Build history of the part. All positions in model axes, mm. Face numbers are marked on the shaded views. A direction names the side the tool comes from. Round coordinates to 2 decimals unless told otherwise and drop trailing zeros. Order: outer loops, then holes, each group sorted by start corner. A loop starts at its lowest first (then second) coordinate and runs counter-clockwise, first axis right, second up. Notation, with made-up numbers: (42, 38) -> (97, 38) arc R34 cw to (97, 73) -> close; hole circle Ø10 at (17, 19). An arc over 180 degrees is marked (long way). Write item = value, one per line.
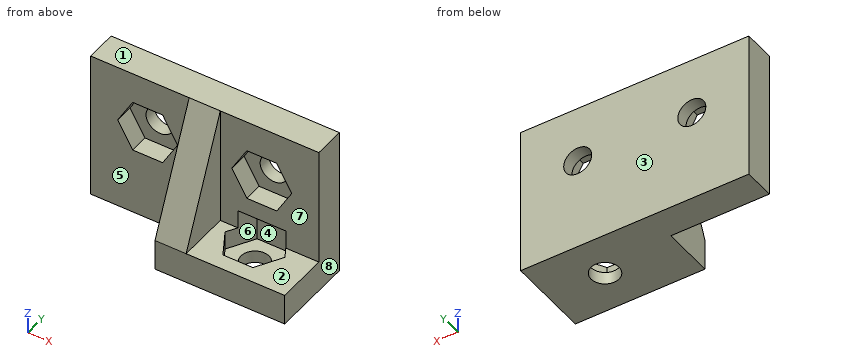
from build123d import *

# Parameters (mm, degrees)
EXTRUDE003_DEPTH  = 3.6
CYLINDER002_R     = 1.35
CYLINDER002_DEPTH = 3
EXTRUDE002_DEPTH  = 1.8
CYLINDER003_R     = 1.35
CYLINDER003_DEPTH = 30
EXTRUDE001_DEPTH  = 1.8
CYLINDER_R        = 1.35
CYLINDER_DEPTH    = 3
BOX_W             = 22
BOX_H             = 3
BOX_DEPTH         = 14.5
BOX001_W          = 12.5
BOX001_H          = 5
BOX001_DEPTH      = 3
EXTRUDE_DEPTH     = 3


with BuildPart() as extrude003:
    # Sketch003 → Extrude003 (new body)
    with BuildSketch(Plane.XY):
        Polygon((2.8868, 0), (1.4434, 2.500042), (-1.4434, 2.500042), (-2.8868, 0), (-1.4434, -2.500042), (1.4434, -2.500042), align=None)
    extrude(amount=EXTRUDE003_DEPTH)


with BuildPart() as extrude003_1:
    # Extrude003 placement: moved
    add(extrude003.part.moved(Location((16.5, -1, 1.2))))


with BuildPart() as hole03:
    # Cylinder002 → Cylinder002 (new body)
    with BuildSketch(Plane(origin=(16.5, -1, 0), x_dir=(0, 1, 0), z_dir=(0, 0, 1))):
        Circle(CYLINDER002_R)
    extrude(amount=CYLINDER002_DEPTH)

    # Fusion002: union Extrude003
    add(extrude003_1.part)


with BuildPart() as extrude002:
    # Sketch002 → Extrude002 (new body)
    with BuildSketch(Plane(origin=(16.5, 1.8, 9), x_dir=(1, 0, 0), z_dir=(0, -1, 0))):
        Polygon((2.8868, 0), (1.4434, 2.500042), (-1.4434, 2.500042), (-2.8868, 0), (-1.4434, -2.500042), (1.4434, -2.500042), align=None)
    extrude(amount=EXTRUDE002_DEPTH)


with BuildPart() as hole02:
    # Cylinder003 → Cylinder003 (new body)
    with BuildSketch(Plane(origin=(16.5, 3, 9), x_dir=(1, 0, 0), z_dir=(0, -1, 0))):
        Circle(CYLINDER003_R)
    extrude(amount=CYLINDER003_DEPTH)

    # Fusion001: union Extrude002
    add(extrude002.part)


with BuildPart() as extrude001:
    # Sketch001 → Extrude001 (new body)
    with BuildSketch(Plane(origin=(5.5, 1.8, 9), x_dir=(1, 0, 0), z_dir=(0, -1, 0))):
        Polygon((2.8868, 0), (1.4434, 2.500042), (-1.4434, 2.500042), (-2.8868, 0), (-1.4434, -2.500042), (1.4434, -2.500042), align=None)
    extrude(amount=EXTRUDE001_DEPTH)


with BuildPart() as hole01:
    # Cylinder → Cylinder (new body)
    with BuildSketch(Plane(origin=(5.5, 3, 9), x_dir=(1, 0, 0), z_dir=(0, -1, 0))):
        Circle(CYLINDER_R)
    extrude(amount=CYLINDER_DEPTH)

    # Fusion: union Extrude001
    add(extrude001.part)


with BuildPart() as cut001:
    # Box → Box (new body)
    with BuildSketch(Plane.XY):
        with Locations((11, 1.5)):
            Rectangle(BOX_W, BOX_H)
    extrude(amount=BOX_DEPTH)

    # Cut: cut Hole01
    add(hole01.part, mode=Mode.SUBTRACT)

    # Cut001: cut Hole02
    add(hole02.part, mode=Mode.SUBTRACT)


with BuildPart() as cut002:
    # Box001 → Box001 (new body)
    with BuildSketch(Plane(origin=(9.5, -5, 0), x_dir=(1, 0, 0), z_dir=(0, 0, 1))):
        with Locations((6.25, 2.5)):
            Rectangle(BOX001_W, BOX001_H)
    extrude(amount=BOX001_DEPTH)

    # Fusion003: union Cut001
    add(cut001.part)

    # Cut002: cut Hole03
    add(hole03.part, mode=Mode.SUBTRACT)


with BuildPart() as left_hand_bracket:
    # Sketch → Extrude (new body)
    with BuildSketch(Plane(origin=(0, 0, 1.4), x_dir=(0, 1, 0), z_dir=(1, 0, 0))):
        Polygon((0, 11.5), (0, 0), (-5, 0), align=None)
    extrude(amount=EXTRUDE_DEPTH)


with BuildPart() as left_hand_bracket_1:
    # Extrude placement: moved
    add(left_hand_bracket.part.moved(Location((9.5, 0, 1.6))))

    # Fusion004: union Cut002
    add(cut002.part)


solid = left_hand_bracket_1.part
Q1. Cut at C-C, the plane x = 16.5. List the corners of the cut face in (y, z), and give its area (3 significant figures).
Check values:
outline = (-5, 0) -> (-2.35, 0) -> (-2.35, 1.2) -> (-3.5, 1.2) -> (-3.5, 3) -> (-5, 3) -> close; (0, 4.8) -> (1.5, 4.8) -> (1.5, 1.2) -> (0.35, 1.2) -> (0.35, 0) -> (3, 0) -> (3, 7.65) -> (1.8, 7.65) -> (1.8, 6.5) -> (0, 6.5) -> close; (0, 11.5) -> (1.8, 11.5) -> (1.8, 10.35) -> (3, 10.35) -> (3, 14.5) -> (0, 14.5) -> close
area = 31.3 mm²
Q2. Cut at A-A, the plane x = 5.5. List the corners of the cut face in (y, z), and give its area (3 significant figures).
Check values:
outline = (0, 0) -> (3, 0) -> (3, 7.65) -> (1.8, 7.65) -> (1.8, 6.5) -> (0, 6.5) -> close; (0, 11.5) -> (1.8, 11.5) -> (1.8, 10.35) -> (3, 10.35) -> (3, 14.5) -> (0, 14.5) -> close
area = 31.3 mm²
Q3. Cut at B-B, the plane y = 2.5. List the corners of the cut face in (x, z).
Check values:
outline = (0, 0) -> (22, 0) -> (22, 14.5) -> (0, 14.5) -> close; hole circle Ø2.7 at (5.5, 9); hole circle Ø2.7 at (16.5, 9)
Q4. Mould opens along Y. For the marked faces 6, 7 and 8 say: released by +Y, released by -Y, zero draft, split by the parting line, or undercut.
Check values:
face_6 = undercut
face_7 = released by -Y
face_8 = zero draft
Q5. Probe probe 1 along X at (y, z) = (2.35, 9); probe 2 along Z at (x, y) = (5.5, 2.7); probe 3 along Y at (x, z) = (7.5, 13). List the from-to ranges inside material, lowest first.
Check values:
probe_1 = 0 to 4.15, 6.85 to 15.15, 17.85 to 22
probe_2 = 0 to 7.65, 10.35 to 14.5
probe_3 = 0 to 3
Q6. Flat gauge pins, fed straight in: pin 1 (7.5 mm diameter, centred on x = 5.5, z = 9.5, fed in from -Y); pin 2 (1.6 mm diameter, centred on x = 16.5, z = 9, fed in from +Y); pin 3 (1.5 mm diameter, centred on y = -3, z = 7, fed in from -X); pin 4 (1 mm diameter, centred on x = 18, y = -1, fed in from +Z). Where does each tip first touch, or does it go through?
Check values:
pin_1 = 0
pin_2 = through
pin_3 = 9.5
pin_4 = 1.2
Q7. Cut at D-D, the plane y = -0.5. List the corners of the cut face in (x, z), and give its area (3 significant figures).
Check values:
outline = (9.5, 0) -> (15.25, 0) -> (15.25, 1.2) -> (13.9, 1.2) -> (13.9, 3) -> (12.5, 3) -> (12.5, 13.35) -> (9.5, 13.35) -> close; (17.75, 0) -> (22, 0) -> (22, 3) -> (19.1, 3) -> (19.1, 1.2) -> (17.75, 1.2) -> close
area = 56.2 mm²
Q8. Which spindle directions (+Z, -Z, +X, -X, +Y, -Y) get a long thin tool onto all of the face, cutting with end or side? Do the marked faces 1, 2, 3, 4 and 5. Say none if no direction does.
Check values:
face_1 = +Z, +X, -X, +Y, -Y
face_2 = +Z, +X, -Y
face_3 = +Z, -Z, +X, -X, +Y
face_4 = none
face_5 = +Z, -Z, -X, -Y
